Here's how the part is built. I have some questions about the finished solid (model axes, mm). A direction names the side the tool comes from. Round coordinates to 2 decimals unless told otherwise and drop trailing zeros. Write each loop counter-clockwise with the first axis right and the second up, starting at its lowest first coordinate (ties: lowest second). Pieces come first, ordered by that corner, then holes. Notation, with made-up numbers: (-9, 6) - (20, 6) arc R32 cw to (20, 37) - close; hole circle Ø10 at (-17, 54.25). An arc over 180 degrees is marked (long way). Write item = value, one per line. Start each with the question number.
Item 1: For P1, Ø1.5, axis at x = -8, z = -1, coming from the -Y side; P2, Ø6.5, axis at x = 3, y = 3, coming from the +Z side; P3, Ø6, axis at x = -3.5, y = -8.5, coming from the +Z side, each with a flat end and sliding along its axis, tell me the tip position at first contact or that it passes through.
Item 2: If I drill on line 1 along X through (y, z) = (-4.5, 4.5); line 2 along Y through (x, z) = (2.5, 3), over which ranges is the centre line in solid material (lowest first)? Write a range as [from, to].
Item 3: Which directions (+Z, -Z, +X, -X, +Y, -Y) give clear straight access to the entire face, cutting with the end or side of a thin tool? Please do faces 4 (the face through (0, 0, -2)), 5 (the face through (12.4, 0.15, 0.57)).
Item 4: Thinking about a two-plate mould opening in X: for faces 1 (the face through (0, 2.085, 4)), 2 (the face through (-0.18, -14.4, -1.43)), 3 (the face through (14.4, 14.43, 4.19)), which applies, pulls with the +X half, pulls with the -X half, needs draft (parallel to the pull), parting line crosses it, or undercut?
Item 5: If we section it at C-C (z = 4.5): Give the number of separate pieces and of enclosed holes in the cut face, and give its area (3 significant figures).
Item 6: If we section it at A-A (y = -8.5): Please give me the cut outline in (x, z).
```python
from build123d import *

# Parameters (mm, degrees)
EXTRUDE_1_DEPTH = 8.5
SKETCH_1_6_R    = 2.7
EXTRUDE_2_DEPTH = 8
EXTRUDE_START   = -2
EXTRUDE_3_DEPTH = 2
FILLET_1_R      = 2
CHAMFER_1_SIZE  = 0.2
FILLET_2_R      = 2
FILLET_3_SIZE   = 5
FILLET_3_SIZE_2 = 5.5


with BuildPart() as part:
    # Sketch 1 → Extrude 1 (new body)
    with BuildSketch(Plane.XY):
        with BuildLine():
            ThreePointArc((-15, 13), (-14.414213562, 14.414213562), (-13, 15))
            Line((-13, 15), (13, 15))
            ThreePointArc((13, 15), (14.414213562, 14.414213562), (15, 13))
            Line((15, 13), (15, -13))
            ThreePointArc((15, -13), (14.414213562, -14.414213562), (13, -15))
            Line((13, -15), (-13, -15))
            ThreePointArc((-13, -15), (-14.414213562, -14.414213562), (-15, -13))
            Line((-15, -13), (-15, 13))
        make_face()
        with BuildLine():
            ThreePointArc((-13, -11), (-12.414213562, -12.414213562), (-11, -13))
            Line((-11, -13), (11, -13))
            ThreePointArc((11, -13), (12.414213562, -12.414213562), (13, -11))
            Line((13, -11), (13, 11))
            ThreePointArc((13, 11), (12.414213562, 12.414213562), (11, 13))
            Line((11, 13), (-11, 13))
            ThreePointArc((-11, 13), (-12.414213562, 12.414213562), (-13, 11))
            Line((-13, 11), (-13, -11))
        make_face(mode=Mode.SUBTRACT)
    extrude(amount=EXTRUDE_1_DEPTH)



with BuildPart() as body_2:
    # Sketch 1_6 → Extrude 2 (new body)
    with BuildSketch(Plane.XY):
        Circle(SKETCH_1_6_R)
        Polygon((-2.085, -0.585), (-2.085, 0.585), (-0.585, 0.585), (-0.585, 2.085), (0.585, 2.085), (0.585, 0.585), (2.085, 0.585), (2.085, -0.585), (0.585, -0.585), (0.585, -2.085), (-0.585, -2.085), (-0.585, -0.585), align=None, mode=Mode.SUBTRACT)
    extrude(amount=EXTRUDE_2_DEPTH)


with BuildPart() as part_1:
    add(part.part)

    add(body_2.part)  # Extrude 3 merges body 2
    # Sketch 1_7 → Extrude 3 (add)
    with BuildSketch(Plane.XY.offset(EXTRUDE_START)):
        with BuildLine():
            Line((-13, 15), (13, 15))
            ThreePointArc((13, 15), (14.414213562, 14.414213562), (15, 13))
            Line((15, 13), (15, -13))
            ThreePointArc((15, -13), (14.414213562, -14.414213562), (13, -15))
            Line((13, -15), (-13, -15))
            ThreePointArc((-13, -15), (-14.414213562, -14.414213562), (-15, -13))
            Line((-15, -13), (-15, 13))
            ThreePointArc((-15, 13), (-14.414213562, 14.414213562), (-13, 15))
        make_face()
    extrude(amount=EXTRUDE_3_DEPTH)

    # Fillet 1
    fillet_1_edges = [part_1.edges().sort_by_distance(p)[0] for p in [
        (-14.414213562, -14.414213562, -2),
        (-15, 0, -2),
        (14.414213562, 14.414213562, -2),
        (14.414213562, -14.414213562, -2),
        (0, -15, -2),
        (-14.414213562, 14.414213562, -2),
        (0, 15, -2),
        (15, 0, -2),
    ]]
    fillet(fillet_1_edges, radius=FILLET_1_R)

    # Chamfer 1
    chamfer_1_edges = [part_1.edges().sort_by_distance(p)[0] for p in [
        (1.335, -0.585, 8),
        (0, -2.085, 8),
        (-0.585, -1.335, 8),
        (-1.335, -0.585, 8),
        (-2.085, 0, 8),
        (-0.585, 1.335, 8),
        (0, 2.085, 8),
        (0.585, 1.335, 8),
        (1.335, 0.585, 8),
        (2.085, 0, 8),
        (0.585, -1.335, 8),
        (-1.335, 0.585, 8),
    ]]
    chamfer(chamfer_1_edges, length=CHAMFER_1_SIZE)

    # Fillet 2
    fillet_2_edges = [part_1.edges().sort_by_distance(p)[0] for p in [
        (0, -13, 0),
        (12.414213562, -12.414213562, 0),
        (13, 0, 0),
        (12.414213562, 12.414213562, 0),
        (0, 13, 0),
        (-12.414213562, 12.414213562, 0),
        (-13, 0, 0),
        (-12.414213562, -12.414213562, 0),
    ]]
    fillet(fillet_2_edges, radius=FILLET_2_R)

    # Fillet 3
    # a fillet whose section is not a circle: 5.5, 5 mm, written as the material it adds along each edge
    with BuildSketch(Plane(origin=(0, 0, 0), x_dir=(1, 0, 0), z_dir=(0, -1, 0))) as fillet_3_piece_1:
        with BuildLine():
            Bezier((2.7 + FILLET_3_SIZE, 0), (2.7, 0), (2.7, FILLET_3_SIZE_2), weights=[1, 0.333333333, 1])
            Line((2.7, FILLET_3_SIZE_2), (2.7, 0))
            Line((2.7, 0), (2.7 + FILLET_3_SIZE, 0))
        make_face()
    revolve(axis=Axis((0, 0, 0), (0, 0, 1)))


solid = part_1.part
```
Reply:
q1.P1 = -14.98
q1.P2 = 8
q1.P3 = 0.63
q2.line_1 = [-15, -13], [13, 15]
q2.line_2 = [-15, -13], [-2.88, 2.88], [13, 15]
q3.face_4 = -Z, +X, -X, +Y, -Y
q3.face_5 = +Z
q4.face_1 = undercut
q4.face_2 = needs draft
q4.face_3 = pulls with the +X half
q5.separate_pieces = 2
q5.enclosed_holes = 2
q5.area = 243 mm2
q6.outline = (-15, 0) arc R2 ccw to (-13, -2) - (13, -2) arc R2 ccw to (15, 0) - (15, 8.5) - (13, 8.5) - (13, 2) arc R2 cw to (11, 0) - (-11, 0) arc R2 cw to (-13, 2) - (-13, 8.5) - (-15, 8.5) - close
